Could you check a few things on this model? Use its own coordinates, in mm. A direction names the side the tool comes from. Give positions to 0.01 mm unless a question says otherwise; leave off trailing zeros. Order: outer loops, then holes, each group sorted by start corner. A loop starts at its lowest first (then second) coordinate and runs counter-clockwise, first axis right, second up.
(1) Imagine slicing it at C-C, the plane z = -19. Write out the boundary of the cut face in (x, y), then the cut area to 3 significant figures.
(2) On a 3-axis mill with a long thin cutter (end or side, diameter ignored), from which of +Z, -Z, +X, -X, +Y, -Y can I reach the whole of each face in a straight line? I mean faces 4 (the flat face through (15, -28, 0)), 5 (the cylindrical face through (23.1, -28.53, 17.93)), 6 (the cylindrical face through (13.476, -0.632, 28.531)), 7 (the flat face through (-23, -25.4, 0)). Say none if no direction works.
(3) Imagine slicing it at D-D, the plane x = -22.5. Write out the boundary of the cut face in (y, z), then the cut area to 3 significant figures.
(4) Imagine slicing it at A-A, the plane y = 12. Write out the boundary of the cut face in (x, z), then the cut area to 3 significant figures.
(5) If we mould it in two halves opening along Y, with no side actions, what happens to faces 1 (the flat face through (7, 8, -31.75)), 2 (the flat face through (0, -16.75, -29)), 3 (the flat face through (0, 25.4, 0))? For each: released by +Y, released by -Y, zero draft, split by the parting line, or undercut.
(6) Imagine slicing it at B-B, the plane x = 18. Write out the boundary of the cut face in (y, z), then the cut area to 3 significant figures.
(7) Will these pins go through, and if not, where does the flat tip stop? pin 1 (9.5 mm diameter, centred on x = 23.75, z = 15, fed in from -Y); pin 2 (3 mm diameter, centred on x = -4.5, z = 28, fed in from -Y); pin 3 (8 mm diameter, centred on y = -18, z = 10.5, fed in from -X).
(8) If I drill on probe 1 along X at (y, z) = (-30.25, -15); probe 2 along Z at (x, y) = (23.75, -27); probe 3 along Y at (x, z) = (-24.5, 21.5), over which ranges is the centre line in solid material (lowest first)?
from build123d import *

# Parameters (mm, degrees)
SKETCH1_W                 = 63.5
SKETCH1_H                 = 63.5
BOSS_EXTRUDE1_DEPTH       = 31.75
SHELL1_T                  = -6.35
SKETCH2_W                 = 30
SKETCH2_H                 = 15
CUT_EXTRUDE1_DEPTH        = 32.75
CUT_EXTRUDE1_DEPTH_BACK   = 32.75
SKETCH3_R                 = 6
CUT_EXTRUDE2_DEPTH        = 32.75
M4X0_7_TAPPED_HOLE3_D     = 3.3
M4X0_7_TAPPED_HOLE3_DEPTH = 6.35
SKETCH8_R                 = 9
SKETCH8_R_2               = 2
CUT_EXTRUDE3_DEPTH        = 32.75
SKETCH9_R                 = 3
CUT_EXTRUDE4_DEPTH        = 32.75


with BuildPart() as part:
    # Sketch1 → Boss-Extrude1 (new body, symmetric)
    with BuildSketch(Plane(origin=(0, 0, 0), x_dir=(1, 0, 0), z_dir=(0, 1, 0))):
        Rectangle(SKETCH1_W, SKETCH1_H)
    extrude(amount=BOSS_EXTRUDE1_DEPTH, both=True)

    # Shell1
    shell1_openings = [part.faces().sort_by_distance(p)[0] for p in [
        (-31.75, 0, 0),
        (31.75, 0, 0),
    ]]
    offset(amount=SHELL1_T, openings=shell1_openings, kind=Kind.INTERSECTION)

    # Sketch2 → Cut-Extrude1 (cut, two sides)
    with BuildSketch(Plane.XY) as cut_extrude1_sk:
        with Locations((0, -24.25)):
            Rectangle(SKETCH2_W, SKETCH2_H)
    extrude(amount=CUT_EXTRUDE1_DEPTH, mode=Mode.SUBTRACT)
    extrude(cut_extrude1_sk.sketch, amount=-CUT_EXTRUDE1_DEPTH_BACK, mode=Mode.SUBTRACT)

    # Sketch3 → Cut-Extrude2 (cut, through all)
    with BuildSketch(Plane.XY):
        Circle(SKETCH3_R)
    extrude(amount=CUT_EXTRUDE2_DEPTH, mode=Mode.SUBTRACT)

    # M4x0.7 Tapped Hole3
    with Locations(Plane(origin=(-15, 0, 31.75), x_dir=(1, 0, 0), z_dir=(0, 0, 1))):
        with Locations((0, 0), (30, 0)):
            Hole(M4X0_7_TAPPED_HOLE3_D / 2, depth=M4X0_7_TAPPED_HOLE3_DEPTH)

    # Sketch8 → Cut-Extrude3 (cut, through all)
    with BuildSketch(Plane.XY):
        Circle(SKETCH8_R)
        with Locations((-14, 7)):
            Circle(SKETCH8_R_2)
        with Locations((14, 7)):
            Circle(SKETCH8_R_2)
    extrude(amount=-CUT_EXTRUDE3_DEPTH, mode=Mode.SUBTRACT)

    # Sketch9 → Cut-Extrude4 (cut, through all)
    with BuildSketch(Plane(origin=(0, 0, 0), x_dir=(1, 0, 0), z_dir=(0, 1, 0))):
        with Locations((-23.75, -15)):
            Circle(SKETCH9_R)
        with Locations((23.75, -15)):
            Circle(SKETCH9_R)
        with Locations((23.75, 15)):
            Circle(SKETCH9_R)
        with Locations((-23.75, 15)):
            Circle(SKETCH9_R)
    extrude(amount=-CUT_EXTRUDE4_DEPTH, mode=Mode.SUBTRACT)


solid = part.part
Answer block:
1. outline: (-31.75, -31.75) - (-15, -31.75) - (-15, -25.4) - (-31.75, -25.4) - close; (-31.75, 25.4) - (31.75, 25.4) - (31.75, 31.75) - (-31.75, 31.75) - close; (15, -31.75) - (31.75, -31.75) - (31.75, -25.4) - (15, -25.4) - close
1. area: 616 mm2
2. face 4: +Z, -Z, -Y
2. face 5: -Y
2. face 6: +Z
2. face 7: +X, -X
3. outline: (-31.75, -31.75) - (31.75, -31.75) - (31.75, 31.75) - (-31.75, 31.75) - (-31.75, 17.73) - (-25.4, 17.73) - (-25.4, 25.4) - (25.4, 25.4) - (25.4, -25.4) - (-25.4, -25.4) - (-25.4, -17.73) - (-31.75, -17.73) - close; (-31.75, -12.27) - (-25.4, -12.27) - (-25.4, 12.27) - (-31.75, 12.27) - close
3. area: 1,380 mm2
4. outline: (-31.75, -31.75) - (31.75, -31.75) - (31.75, -25.4) - (-31.75, -25.4) - close; (-31.75, 25.4) - (31.75, 25.4) - (31.75, 31.75) - (-31.75, 31.75) - close
4. area: 806 mm2
5. face 1: zero draft
5. face 2: released by -Y
5. face 3: undercut
6. outline: (-31.75, -31.75) - (31.75, -31.75) - (31.75, 31.75) - (-31.75, 31.75) - close; hole (-25.4, -25.4) - (25.4, -25.4) - (25.4, 25.4) - (-25.4, 25.4) - close
6. area: 1,450 mm2
7. pin 1: stops at y = -31.75
7. pin 2: stops at y = -16.75
7. pin 3: passes through
8. probe 1: x = -31.75 to -26.75, -20.75 to -15, 15 to 20.75, 26.75 to 31.75
8. probe 2: z = -31.75 to -18, -12 to 12, 18 to 31.75
8. probe 3: y = -31.75 to -25.4, 25.4 to 31.75
